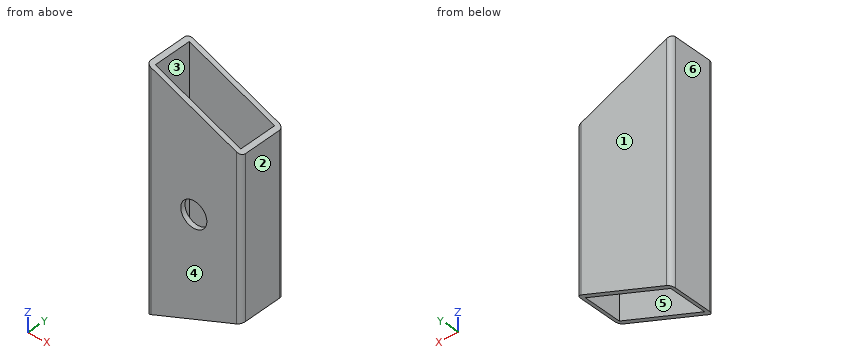
Autodesk Inventor part; units mm, degrees
ref_plane "YZ Plane" through (0, 0, 0) normal (1, 0, 0) x (0, 1, 0)
ref_plane "XZ Plane" through (0, 0, 0) normal (0, 1, 0) x (-1, 0, 0)
ref_plane "XY Plane" through (0, 0, 0) normal (0, 0, 1) x (1, 0, 0)
sketch "Sketch1" plane through (0, 0, 0) normal (0, 0, 1) x (1, 0, 0)
  line L0 (-20, 10) -> (20, 10)
  line L1 (20, 10) -> (20, -10)
  line L2 (20, -10) -> (-20, -10)
  line L3 (-20, -10) -> (-20, 10)
  line L4 (-20, 10) -> (20, -10) construction
  line L5 (20, 10) -> (-20, -10) construction
  line L6 (18, 8) -> (-18, 8)
  line L7 (-18, 8) -> (-18, -8)
  line L8 (-18, -8) -> (18, -8)
  line L9 (18, -8) -> (18, 8)
  point P0 (0, 0)
  dimension "d0" = 40
  dimension "d1" = 20
  dimension "d2" = 2
extrude "Extrusion1" add sketch "Sketch1" along normal mid plane 100
sketch "Sketch2" plane through (0, 0, 0) normal (0, 1, 0) x (-1, 0, 0)
  line L0 (20, -50) -> (20, 50)
  line L1 (-20, 50) -> (20, 50)
  line L2 (-20, -50) -> (-20, 50)
  line L3 (20, -50) -> (-20, -50)
  line L4 (20, -50) -> (-20, -33.4315)
  line L5 (-20, -50) -> (-20, 50)
  point P0 (0, 0)
  dimension "d20" = 22.5
extrude "Extrusion2" cut sketch "Sketch2" along normal through all both and the other way through all contours L3 L2 L4
mirror "Mirror1" about plane through (0, 0, 0) normal (0, 0, 1) of "Extrusion2"
fillet "Fillet1" radius 2 4 edges at (-20, 10, 0) (-20, -10, 0) (20, -10, 0) (20, 10, 0)
sketch "Sketch4" plane through (0, 0, 0) normal (0, 1, 0) x (-1, 0, 0)
  circle A0 centre (0, 0) radius 5.5
  dimension "d21" = 11
extrude "Extrusion4" cut sketch "Sketch4" against normal through all
properties part number "Short tube 2"
Here's how the part is built. I have some questions about the finished solid (model axes, mm). Face numbers are marked on the shaded views. A direction names the side the tool comes from. Give positions to 0.01 mm unless a question says otherwise; leave off trailing zeros. Write each loop counter-clockwise with the first axis right and the second up, starting at its lowest first coordinate (ties: lowest second). Pieces come first, ordered by that corner, then holes. Notation, with made-up numbers: (11, 13.25) -> (35, 13.25) arc R13 cw to (35, 18.25) -> close; hole circle Ø11 at (46, 30.25). An arc over 180 degrees is marked (long way). Use one line per item in the form item = value.
1) Suppose I cut it at B-B (z = 8). Please give me the cut outline in (x, y), and give its area (3 significant figures).
Verdict:
outline = (-20, -8) arc R2 ccw to (-18, -10) -> (18, -10) arc R2 ccw to (20, -8) -> (20, 8) arc R2 ccw to (18, 10) -> (-18, 10) arc R2 ccw to (-20, 8) -> close; hole (-18, -8) -> (18, -8) -> (18, 8) -> (-18, 8) -> close
area = 221 mm2
2) We'd pull the mould along Y, two halves only. Please class the marked faces 1, 2, 3 and 4: +Y half, -Y half, draft (parallel to the pull), parting line (faces both ways), or undercut.
Verdict:
face_1 = +Y half
face_2 = draft
face_3 = undercut
face_4 = -Y half
3) Suppose I cut it at D-D (x = 1). Please give me the cut outline in (y, z).
Verdict:
outline = (-10, -41.3) -> (-8, -41.3) -> (-8, -5.41) -> (-10, -5.41) -> close; (-10, 5.41) -> (-8, 5.41) -> (-8, 41.3) -> (-10, 41.3) -> close; (8, -41.3) -> (10, -41.3) -> (10, 41.3) -> (8, 41.3) -> close
4) Suppose I cut it at C-C (x = 7.5). Please give me the cut outline in (y, z).
Verdict:
outline = (-10, -38.61) -> (-8, -38.61) -> (-8, 38.61) -> (-10, 38.61) -> close; (8, -38.61) -> (10, -38.61) -> (10, 38.61) -> (8, 38.61) -> close
5) On a 3-axis mill with a long thin cutter (end or side, diameter ignored), from which of +Z, -Z, +X, -X, +Y, -Y can I reach the whole of each face in a straight line? I mean the marked faces 5 and 6. Say none if no direction works.
Verdict:
face_5 = +Z, -Z
face_6 = +Z, -Z, -X, +Y, -Y
6) If I drill on L1, parallel to Y at x = -6.5, z = 33; L2, parallel to X at y = -7, z = 13; L3, parallel to X at y = -6, z = 38.5, over which ranges is the centre line in solid material (lowest first)? Write a range as [from, to].
Verdict:
L1 = [-10, -8], [8, 10]
L2 = [-20, -18], [18, 20]
L3 = [-20, -18]
7) Suppose I cut it at A-A (y = 5.5). Please give me the cut outline in (x, z).
Verdict:
outline = (-20, -50) -> (-18, -49.17) -> (-18, 49.17) -> (-20, 50) -> close; (18, -34.26) -> (20, -33.43) -> (20, 33.43) -> (18, 34.26) -> close
